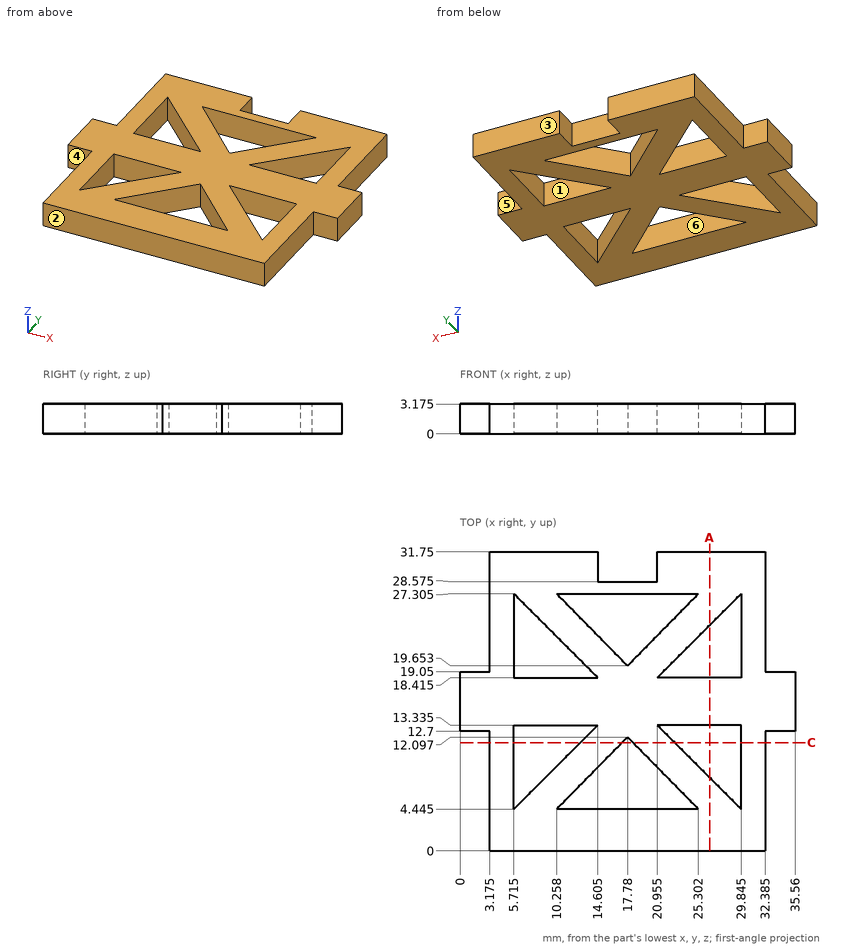
Could you check a few things on this drawing? It's one solid part, dimensions in mm from its lowest x, y, z. A direction names the side the tool comes from. Give positions to 0.01 mm unless a question says otherwise; leave off trailing zeros. Write each loop counter-clockwise with the first axis right and the second up, starting at its lowest first coordinate (ties: lowest second). Pieces come first, ordered by that corner, then holes. Notation, with made-up numbers: M 16.5,-35 L 26.5,-35 A10 ccw 26.5,-20 Z; hole C 88,29.5 d10. An arc over 180 degrees is marked long. Put each result on its own line as item: value. Start each with the question number.
Item 1: On a 3-axis mill with a long thin cutter (end or side, diameter ignored), from which of +Z, -Z, +X, -X, +Y, -Y can I reach the whole of each face in a straight line? I mean the marked faces 4, 5 and 6. Say none if no direction works.
Item 2: If we section it at A-A, the plane x = 26.5: Count the separate pieces of the cut face and the enclosed holes in it, then the cut area to 3 significant figures.
Item 3: I need wall thicknesses on L1, parallel to X at y = 6.5, z = 1.65 (1 decimal); L2, parallel to Y at x = 20, z = 1.6 (1 decimal); L3, parallel to X at y = 12, z = 1.3 (1 decimal). Which ranges of each line are inside material? Lowest first, please. Write a range as from..to.
Item 4: Thinking about a two-plate mould opening in Y: for the marked faces 1, 2 and 3, which applies, +Y half, -Y half, draft (parallel to the pull), parting line (faces both ways), or undercut?
Item 5: Will these pins go through, and if not, where does the flat tip stop? pin 1 (1.6 mm diameter, centred on x = 18.5, z = 2.5, fed in from +Y) (3 decimals); pin 2 (1 mm diameter, centred on x = 1.5, z = 2, fed in from -Y); pin 3 (1 mm diameter, centred on y = 24.5, z = 1.5, fed in from -X) (3 decimals).
Item 6: If we section it at C-C, the plane y = 11.5: Write out the boundary of the cut face in (x, z) (1 decimal), then the cut area to 3 significant figures.
Values:
1. face 4: +Z, -Z, -X, -Y
1. face 5: +Z, -Z, +X, +Y
1. face 6: +Z, -Z
2. separate pieces: 3
2. enclosed holes: 0
2. area: 65.6 mm²
3. L1: 3.2..5.7, 7.8..12.3, 23.3..27.8, 29.8..32.4
3. L2: 0..4.4, 9.8..21.9, 27.3..28.6
3. L3: 3.2..5.7, 13.3..17.7, 17.9..22.3, 29.8..32.4
4. face 1: undercut
4. face 2: -Y half
4. face 3: +Y half
5. pin 1: y = 28.575
5. pin 2: y = 12.7
5. pin 3: x = 3.175
6. outline: M 3.2,0 L 5.7,0 L 5.7,3.2 L 3.2,3.2 Z; M 12.8,0 L 17.2,0 L 17.2,3.2 L 12.8,3.2 Z; M 18.4,0 L 22.8,0 L 22.8,3.2 L 18.4,3.2 Z; M 29.8,0 L 32.4,0 L 32.4,3.2 L 29.8,3.2 Z
6. area: 44.2 mm²
